Could you check a few things on this drawing? It's one solid part, dimensions in mm from its lowest x, y, z. Give positions to 0.01 mm unless a question says otherwise; leave off trailing zeros. Loops run counter-clockwise (first coordinate to the right, second up) from the corner with the lowest first, then second, coordinate; pieces in that order, holes last. Notation, with made-up numbers: M 11.5,66.5 L 19.5,66.5 A23 cw 19.5,98.5 Z; hole C 7.25,22 d11. An arc over 180 degrees is marked long. Answer as a JSON object with one key per item and string values.
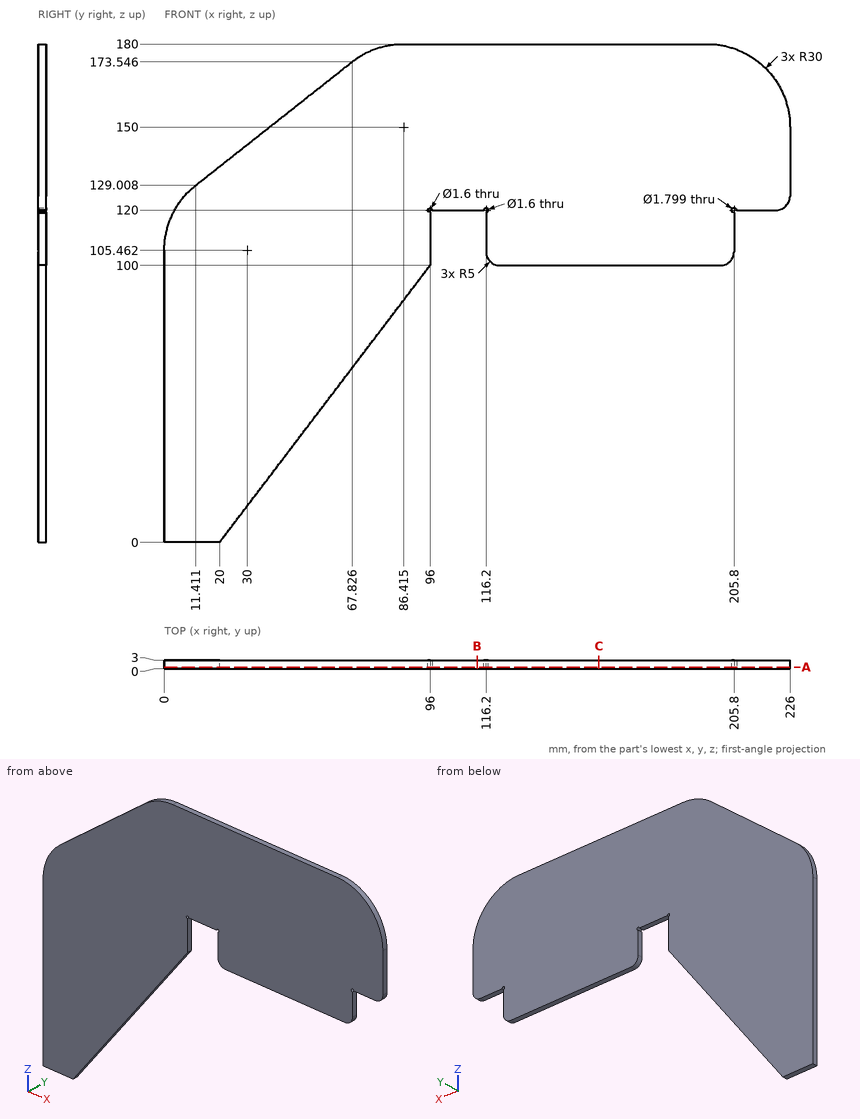
1) Please list where these lines run through material, in increasing order: line 1 along X through (y, z) = (1.35, 105.5); line 2 along Z through (x, y) = (131.5, 2.3); line 3 along Z through (x, y) = (208, 1.35) (1 decimal). Write a range as from..to.
Answer list:
{"line 1": "0..96, 116.2..205.8", "line 2": "100..180", "line 3": "120..177.5"}
2) Suppose I cut it at B-B, the plane x = 113. Write out the boundary of the cut face in (y, z).
Answer list:
{"outline": "M 0,120 L 3,120 L 3,180 L 0,180 Z"}
3) Suppose I cut it at A-A, the plane y = 0.55. Write out the boundary of the cut face in (x, z) (1 decimal), and give its area (3 significant figures).
Answer list:
{"outline": "M 0,0 L 20,0 L 96,100 L 96,119.2 A0.8 cw long 96.8,120 L 115.4,120 A0.8 cw long 116.2,119.2 L 116.2,105 A5 ccw 121.2,100 L 200.8,100 A5 ccw 205.8,105 L 205.8,119.1 A0.9 cw long 206.7,120 L 221,120 A5 ccw 226,125 L 226,150 A30 ccw 196,180 L 86.4,180 A30 ccw 67.8,173.5 L 11.4,129 A30 ccw 0,105.5 Z", "area": "20,500 mm^2"}
4) Suppose I cut it at C-C, the plane x = 157. Write out the boundary of the cut face in (y, z), and give its area (3 significant figures).
Answer list:
{"outline": "M 0,100 L 3,100 L 3,180 L 0,180 Z", "area": "240 mm^2"}
5) Will these pins go through, and if not, where does the flat tip stop? pin 1 Ø1.3 at (x, z) = (116.2, 120) entering from -Y; pin 2 Ø0.9 at (x, y) = (104, 1) entering from -Z; pin 3 Ø1.5 at (y, z) = (2, 110) entering from -X.
Answer list:
{"pin 1": "through", "pin 2": "z = 120", "pin 3": "x = 0.24"}
